The model under review builds one solid part; all positions refer to its coordinate system, in mm. A direction names the side the tool comes from. Give positions to 0.01 mm unless a question says otherwise; leave off trailing zeros. Loops run counter-clockwise (first coordinate to the right, second up) from the corner with the lowest first, then second, coordinate; pieces in that order, holes last. Notation, with made-up numbers: (-21.5, 30) - (27.5, 30) arc R13 ccw to (27.5, 54) - close; hole circle Ø10 at (81, 22). An arc over 180 degrees is marked (long way). Return JSON: item names as keys, results as strings. Group by question number.
```python
from build123d import *

# Parameters (mm, degrees)
ESQUISSE1_R             = 13
BOSS_EXTRU_1_DEPTH      = 6
ESQUISSE2_W             = 12
ESQUISSE2_H             = 6
BOSS_EXTRU_2_DEPTH      = 6
ESQUISSE3_R             = 1.5
ENL_V_MAT_EXTRU_1_DEPTH = 10
ENL_V_MAT_EXTRU_2_DEPTH = 10


with BuildPart() as part:
    # Esquisse1 → Boss.-Extru.1 (new body)
    with BuildSketch(Plane.XY):
        Polygon((55, 13), (53.5, 13), (53.5, 16), (55, 16), (55, 26), (59, 26), (59, 16), (60.5, 16), (60.5, 13), (59, 13), (59, 6), (63, 6), (63, 0), (70, 0), (70, 50), (55, 73.5), (15, 73.5), (0, 50), (0, 0), (7, 0), (7, 6), (11, 6), (11, 13), (9.5, 13), (9.5, 16), (11, 16), (11, 26), (15, 26), (15, 16), (16.5, 16), (16.5, 13), (15, 13), (15, 6), (19, 6), (19, 0), (26, 0), (26, 6), (44, 6), (44, 0), (51, 0), (51, 6), (55, 6), align=None)
        with Locations((35, 33)):
            Circle(ESQUISSE1_R, mode=Mode.SUBTRACT)
    extrude(amount=BOSS_EXTRU_1_DEPTH)

    # Esquisse2 → Boss.-Extru.2 (add)
    with BuildSketch(Plane(origin=(0, 73.5, 0), x_dir=(1, 0, 0), z_dir=(0, 1, 0))):
        with Locations((21, -3)):
            Rectangle(ESQUISSE2_W, ESQUISSE2_H)
        with Locations((49, -3)):
            Rectangle(ESQUISSE2_W, ESQUISSE2_H)
    extrude(amount=BOSS_EXTRU_2_DEPTH)

    # Esquisse3 → Enlèv. mat.-Extru.1 (cut)
    with BuildSketch(Plane.XY.offset(6)):
        with Locations((21.252272915, 23)):
            Circle(ESQUISSE3_R)
        with Locations((48.747727085, 23)):
            Circle(ESQUISSE3_R)
        with Locations((35, 50)):
            Circle(ESQUISSE3_R)
    extrude(amount=-ENL_V_MAT_EXTRU_1_DEPTH, mode=Mode.SUBTRACT)

    # Esquisse4 → Enlèv. mat.-Extru.2 (cut)
    with BuildSketch(Plane.XY.offset(6)):
        Polygon((33, 73.5), (37, 73.5), (37, 67.5), (38, 67.5), (38, 64.5), (37, 64.5), (37, 59.5), (33, 59.5), (33, 64.5), (32, 64.5), (32, 67.5), (33, 67.5), align=None)
    extrude(amount=-ENL_V_MAT_EXTRU_2_DEPTH, mode=Mode.SUBTRACT)


solid = part.part
```
1) We need section B-B, the plane y = 15. Write out the cut boundary in (x, z).
2) To check wall thickness, follow line 1 (X direction, y = 5, z = 3.5); line 2 (Y direction, x = 35, z = 2.2); line 3 (Y direction, x = 54, z = 1.4). State the ranges of each line that lie inside material, in increasing order.
3) We need section C-C, the plane y = 63. Write out the cut boundary in (x, z), plus the area to 3 significant figures.
4) For pin 1 Ø1.8 at (y, z) = (76.5, 4) entering from -X; pin 2 Ø0.5 at (x, z) = (32.5, 2.5) entering from -Y; pin 3 Ø2.5 at (x, y) = (48.75, 23) entering from -Z; pin 4 Ø3 at (y, z) = (58, 2.5) entering from -X, all flat-tipped, find the tip position at first contact; note any pin that passes through.
5) Tool access review of faces 4 (the face through (17, 6, 3)), 5 (the face through (60.5, 15, 3)), 6 (the face through (35, 48, 6)), 7 (the face through (7.6, 61.91, 2.96)), 8 (the face through (35, 59.5, 3)): name each direction out of +Z, -Z, +X, -X, +Y, -Y from which nothing blocks a thin tool from reaching the whole face with its end or side.
6) We need section D-D, the plane z = 2.05. Count the separate pieces of the cut face and the enclosed holes in it, plus the area to 3 significant figures.
7) Draft analysis for pull direction Y (two halves, no side actions). For faces 1 (the face through (15, 10, 3)), 2 (the face through (61, 6, 3)), 3 (the face through (38, 66, 3)), state which applies: +Y half, -Y half, draft (parallel to the pull), parting line (faces both ways), or undercut.
8) We need section A-A, the plane x = 35. Write out the cut boundary in (y, z), plus the area to 3 significant figures.
Findings:
{
 "1": {"outline": "(0, 0) - (9.5, 0) - (9.5, 6) - (0, 6) - close; (16.5, 0) - (53.5, 0) - (53.5, 6) - (16.5, 6) - close; (60.5, 0) - (70, 0) - (70, 6) - (60.5, 6) - close"},
 "2": {"line 1": "x = 0 to 7, 19 to 26, 44 to 51, 63 to 70", "line 2": "y = 6 to 20, 46 to 48.5, 51.5 to 59.5", "line 3": "y = 6 to 13, 16 to 79.5"},
 "3": {"outline": "(8.3, 0) - (33, 0) - (33, 6) - (8.3, 6) - close; (37, 0) - (61.7, 0) - (61.7, 6) - (37, 6) - close", "area": "296 mm^2"},
 "4": {"pin 1": "stops at x = 15", "pin 2": "stops at y = 6", "pin 3": "passes through", "pin 4": "stops at x = 4.15"},
 "5": {"face 4": "+Z, -Z, -Y", "face 5": "+Z, -Z", "face 6": "+Z, +X, -X, +Y, -Y", "face 7": "+Z, -Z, -X, +Y", "face 8": "+Z, -Z, +Y"},
 "6": {"separate pieces": "1", "enclosed holes": "4", "area": "3,890 mm^2"},
 "7": {"face 1": "draft", "face 2": "-Y half", "face 3": "undercut"},
 "8": {"outline": "(6, 0) - (20, 0) - (20, 6) - (6, 6) - close; (46, 0) - (48.5, 0) - (48.5, 6) - (46, 6) - close; (51.5, 0) - (59.5, 0) - (59.5, 6) - (51.5, 6) - close", "area": "147 mm^2"}
}
